from build123d import *

# Parameters (mm, degrees)
SKETCH_1_R      = 1.5
SKETCH_1_R_2    = 2
EXTRUDE_1_DEPTH = 2


with BuildPart() as part:
    # Эскиз1 → Бобышка-Вытянуть1 (new body)
    with BuildSketch(Plane(origin=(0, 0, 0), x_dir=(1, 0, 0), z_dir=(0, 1, 0))):
        with BuildLine():
            Line((-17.625227915, -29.617278809), (12.374772085, -29.617278809))
            Line((12.374772085, -29.617278809), (12.374772085, 48.182721191))
            ThreePointArc((12.374772085, 48.182721191), (-2.625227915, 63.182721191), (-17.625227915, 48.182721191))
            Line((-17.625227915, 48.182721191), (-17.625227915, -29.617278809))
        make_face()
        with Locations(Location((-9.625227915, -24.937945637, 0), (0, 0, 270))):
            Circle(SKETCH_1_R, mode=Mode.SUBTRACT)
        with Locations(Location((4.374772085, -24.937945637, 0), (0, 0, 270))):
            Circle(SKETCH_1_R, mode=Mode.SUBTRACT)
        with Locations(Location((-2.625227915, 48.182721191, 0), (0, 0, 270))):
            Circle(SKETCH_1_R_2, mode=Mode.SUBTRACT)
    extrude(amount=EXTRUDE_1_DEPTH)


solid = part.part
Model file for the job. Use its own axes, mm. Give positions to 0.01 mm unless a question says otherwise; leave off trailing zeros. Order: outer loops, then holes, each group sorted by start corner. A loop starts at its lowest first (then second) coordinate and runs counter-clockwise, first axis right, second up. Notation, with made-up numbers: (52, 58.25) - (96, 58.25) arc R18 ccw to (96, 70.25) - close; hole circle Ø8 at (-25.5, 20). An arc over 180 degrees is marked (long way). One line per item, written item: value.
Item 1: Two-plate mould, pull along Z, no slides. Class faces 1 (the flat face through (-3, 1, 29.617)), 2 (the cylindrical face through (4.44, 0.99, 23.44)), 3 (the cylindrical face through (-9.56, 0.99, 23.44)), 4 (the flat face through (-17.625, 1, -10)): released by +Z, released by -Z, zero draft, split by the parting line, or undercut.
Response values:
face 1: released by +Z
face 2: undercut
face 3: undercut
face 4: zero draft
Item 2: Slice it at C-C (z = -54). List the corners of the cut face in (x, y).
Response values:
outline: (-16.45, 0) - (11.2, 0) - (11.2, 2) - (-16.45, 2) - close
Item 3: Wall check: line 1 (Z direction, x = 5, y = 0.45); line 2 (Z direction, x = -1, y = 0.9); line 3 (X direction, y = 0.35, z = -49.5). Give the ranges that are in metal, low to high.
Response values:
line 1: -61.1 to 23.57, 26.3 to 29.62
line 2: -63.09 to -49.35, -47.02 to 29.62
line 3: -17.57 to -4.13, -1.12 to 12.32
Item 4: Slice it at A-A (y = 1.4). List the corners of the cut face in (x, z).
Response values:
outline: (-17.63, -48.18) arc R15 ccw to (12.37, -48.18) - (12.37, 29.62) - (-17.63, 29.62) - close; hole circle Ø3 at (-9.63, 24.94); hole circle Ø4 at (-2.63, -48.18); hole circle Ø3 at (4.37, 24.94)
Item 5: Slice it at B-B (x = -13.5). List the corners of the cut face in (y, z), then the cut area to 3 significant figures.
Response values:
outline: (0, -58.51) - (2, -58.51) - (2, 29.62) - (0, 29.62) - close
area: 176 mm2
